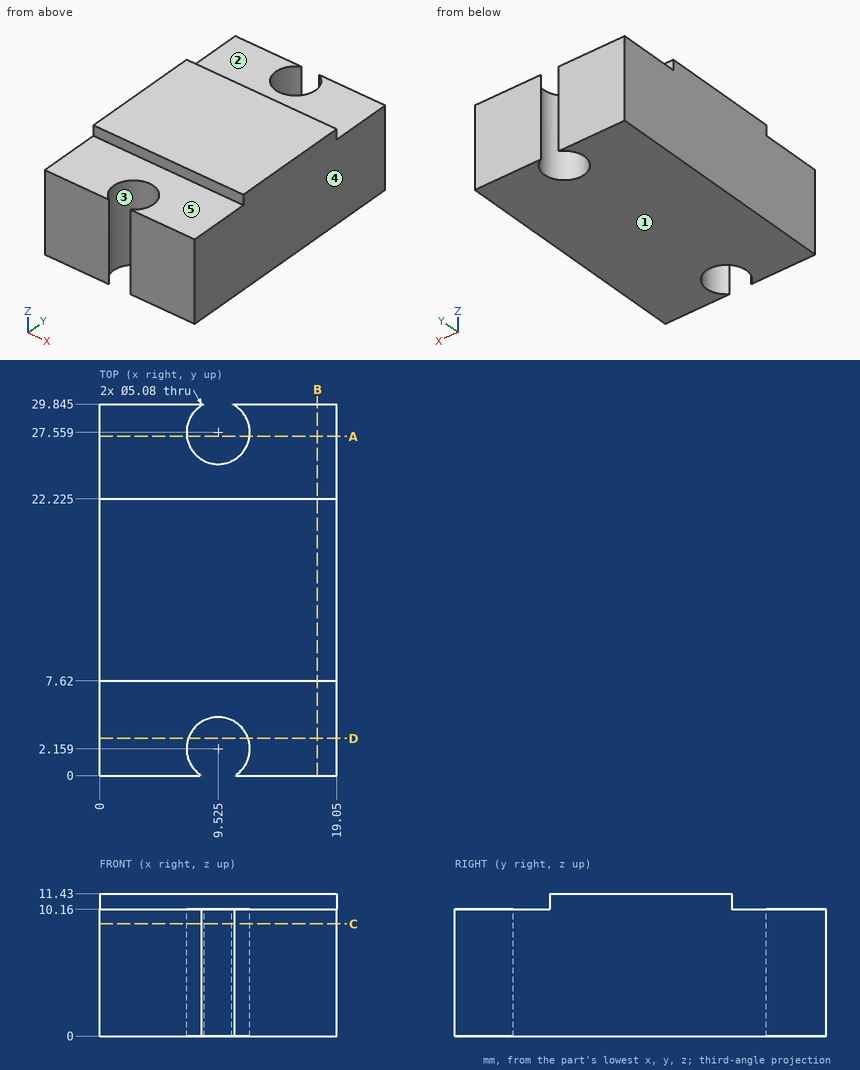
Design review of the part shown in the three views and the two pictorial views. Dimensions are in mm from the part's minimum x, y and z. A direction names the side the tool comes from. Round coordinates to 2 decimals unless told otherwise and drop trailing zeros. Loops run counter-clockwise (first coordinate to the right, second up) from the corner with the lowest first, then second, coordinate; pieces in that order, holes last.
Q1. Add section A-A on y = 27.25. Write out the cut boundary in (x, z).
Result sheet:
outline: (0, 0) - (7, 0) - (7, 10.16) - (0, 10.16) - close; (12.05, 0) - (19.05, 0) - (19.05, 10.16) - (12.05, 10.16) - close
Q2. Mouldability with a two-part tool opening along X and no side actions: class the marked faces 3, 4 and 5 as +X half, -X half, draft (parallel to the pull), parting line (faces both ways), or undercut.
Result sheet:
face 3: undercut
face 4: +X half
face 5: draft
Q3. Add section D-D on y = 3. Write out the cut boundary in (x, z), plus the area to 3 significant figures.
Result sheet:
outline: (0, 0) - (7.13, 0) - (7.13, 10.16) - (0, 10.16) - close; (11.92, 0) - (19.05, 0) - (19.05, 10.16) - (11.92, 10.16) - close
area: 145 mm2
Q4. Insertion check: pin 1 Ø1.4 at (x, z) = (5, 10.5) entering from +Y (3 decimals); pin 2 Ø4 at (x, y) = (9.525, 2.159) entering from +Z; pin 3 Ø1.4 at (x, z) = (6.5, 11) entering from -Y; pin 4 Ø4 at (x, y) = (7, 4) entering from +Z. Each pin has a flat end and moves straight along its axis. Give the tip position at first contact, or say it passes through.
Result sheet:
pin 1: stops at y = 29.845
pin 2: passes through
pin 3: stops at y = 7.62
pin 4: stops at z = 10.16
Q5. Add section B-B on x = 17.5. Write out the cut boundary in (y, z) (3 decimals), plus the area to 3 significant figures.
Result sheet:
outline: (0, 0) - (29.845, 0) - (29.845, 10.16) - (22.225, 10.16) - (22.225, 11.43) - (7.62, 11.43) - (7.62, 10.16) - (0, 10.16) - close
area: 322 mm2
Q6. To check wall thickness, follow line 1 along Y through (x, z) = (7.25, 3.25) (3 decimals); line 2 along Y through (x, z) = (7.5, 5) (3 decimals); line 3 along Y through (x, z) = (7.5, 11) (3 decimals). State the ranges of each line that lie inside material, in increasing order.
Result sheet:
line 1: y = 0 to 1.029, 3.289 to 26.429, 28.689 to 29.845
line 2: y = 0 to 0.626, 3.692 to 26.026, 29.092 to 29.845
line 3: y = 7.62 to 22.225
Q7. Machinability: for the marked faces 1 and 2, which of the approach directions +Z, -Z, +X, -X, +Y, -Y give a long, thin tool a straight path to every point of the face, cutting with its end or side? Answer none if there is none.
Result sheet:
face 1: -Z, +X, -X, +Y, -Y
face 2: +Z, +X, -X, +Y
Q8. Add section C-C on z = 9. Write out the cut boundary in (x, y) (3 decimals), plus the area to 3 significant figures.
Result sheet:
outline: (0, 0) - (8.187, 0) arc R2.54 cw (long way) to (10.863, 0) - (19.05, 0) - (19.05, 29.845) - (10.632, 29.845) arc R2.54 cw (long way) to (8.418, 29.845) - (0, 29.845) - close
area: 529 mm2
